Work out the finished part from the listing and answer in its coordinate system (mm). A direction names the side the tool comes from. Give positions to 0.01 mm unless a question says otherwise; leave off trailing zeros. Write each loop counter-clockwise with the first axis right and the second up, starting at its lowest first coordinate (ties: lowest second). Pieces come first, ordered by that corner, then holes. Notation, with made-up numbers: (-40, -35.5) -> (-7, -35.5) arc R15 ccw to (-7, -14.5) -> close; hole circle Ø3 at (-22.75, 25). An arc over 180 degrees is marked (long way). Write item = value, one per line. Start each with the question number.
from build123d import *

# Parameters (mm, degrees)
SKETCH1_W                      = 128
SKETCH1_H                      = 69
BOSS_EXTRUDE1_DEPTH            = 3
SKETCH5_R                      = 1.55
CUT_EXTRUDE5_DEPTH             = 10
SKETCH7_W                      = 28
SKETCH7_H                      = 8
BOSS_EXTRUDE2_DEPTH            = 5
SKETCH2_R                      = 2.05
CUT_EXTRUDE6_DEPTH             = 73.878323252
CUT_EXTRUDE6_DIRECTION_2_REACH = 74.878
CUT_EXTRUDE7_DEPTH             = 3
SKETCH8_W                      = 18
SKETCH8_H                      = 2
BOSS_EXTRUDE3_DEPTH            = 8
FILLET1_R                      = 3
FILLET2_R                      = 1


with BuildPart() as part:
    # Sketch1 → Boss-Extrude1 (new body)
    with BuildSketch(Plane(origin=(0, 0, 0), x_dir=(1, 0, 0), z_dir=(0, 1, 0))):
        Rectangle(SKETCH1_W, SKETCH1_H)
    extrude(amount=BOSS_EXTRUDE1_DEPTH)

    # Sketch5 → Cut-Extrude5 (cut)
    with BuildSketch(Plane(origin=(0, 3, 0), x_dir=(1, 0, 0), z_dir=(0, 1, 0))):
        with Locations(Location((0, -20.25, 0), (0, 0, 270))):
            Circle(SKETCH5_R)
        with Locations(Location((0, 20.25, 0), (0, 0, 270))):
            Circle(SKETCH5_R)
    extrude(amount=-CUT_EXTRUDE5_DEPTH, mode=Mode.SUBTRACT)

    # Sketch7 → Boss-Extrude2 (add)
    with BuildSketch(Plane(origin=(0, 3, 0), x_dir=(1, 0, 0), z_dir=(0, 1, 0))):
        with Locations((-50, 30.5)):
            Rectangle(SKETCH7_W, SKETCH7_H)
        with Locations((50, 30.5)):
            Rectangle(SKETCH7_W, SKETCH7_H)
        with Locations((50, -30.5)):
            Rectangle(SKETCH7_W, SKETCH7_H)
        with Locations((-50, -30.5)):
            Rectangle(SKETCH7_W, SKETCH7_H)
    extrude(amount=BOSS_EXTRUDE2_DEPTH)

    # Sketch2 → Cut-Extrude6 (cut)
    with BuildSketch(Plane(origin=(0, 3, 0), x_dir=(1, 0, 0), z_dir=(0, 1, 0))):
        with Locations(Location((-45, 30.5, 0), (0, 0, 270))):
            Circle(SKETCH2_R)
        with Locations(Location((45, 30.5, 0), (0, 0, 270))):
            Circle(SKETCH2_R)
        with Locations(Location((45, -30.5, 0), (0, 0, 270))):
            Circle(SKETCH2_R)
        with Locations(Location((-45, -30.5, 0), (0, 0, 270))):
            Circle(SKETCH2_R)
    extrude(amount=-CUT_EXTRUDE6_DEPTH, mode=Mode.SUBTRACT)

    # Sketch2 → Cut-Extrude6 direction 2 (cut, up to next)
    with BuildSketch(Plane(origin=(0, 3, 0), x_dir=(1, 0, 0), z_dir=(0, 1, 0)), mode=Mode.PRIVATE) as cut_extrude6_direction_2_sk1:
        with Locations(Location((-45, 30.5, 0), (0, 0, 270))):
            Circle(SKETCH2_R)
    cut_extrude6_direction_2_tool1 = extrude(cut_extrude6_direction_2_sk1.sketch, amount=CUT_EXTRUDE6_DIRECTION_2_REACH, mode=Mode.PRIVATE) & part.part
    # Sketch2 → Cut-Extrude6 direction 2 (cut, up to next)
    with BuildSketch(Plane(origin=(0, 3, 0), x_dir=(1, 0, 0), z_dir=(0, 1, 0)), mode=Mode.PRIVATE) as cut_extrude6_direction_2_sk2:
        with Locations(Location((45, 30.5, 0), (0, 0, 270))):
            Circle(SKETCH2_R)
    cut_extrude6_direction_2_tool2 = extrude(cut_extrude6_direction_2_sk2.sketch, amount=CUT_EXTRUDE6_DIRECTION_2_REACH, mode=Mode.PRIVATE) & part.part
    # Sketch2 → Cut-Extrude6 direction 2 (cut, up to next)
    with BuildSketch(Plane(origin=(0, 3, 0), x_dir=(1, 0, 0), z_dir=(0, 1, 0)), mode=Mode.PRIVATE) as cut_extrude6_direction_2_sk3:
        with Locations(Location((45, -30.5, 0), (0, 0, 270))):
            Circle(SKETCH2_R)
    cut_extrude6_direction_2_tool3 = extrude(cut_extrude6_direction_2_sk3.sketch, amount=CUT_EXTRUDE6_DIRECTION_2_REACH, mode=Mode.PRIVATE) & part.part
    # Sketch2 → Cut-Extrude6 direction 2 (cut, up to next)
    with BuildSketch(Plane(origin=(0, 3, 0), x_dir=(1, 0, 0), z_dir=(0, 1, 0)), mode=Mode.PRIVATE) as cut_extrude6_direction_2_sk4:
        with Locations(Location((-45, -30.5, 0), (0, 0, 270))):
            Circle(SKETCH2_R)
    cut_extrude6_direction_2_tool4 = extrude(cut_extrude6_direction_2_sk4.sketch, amount=CUT_EXTRUDE6_DIRECTION_2_REACH, mode=Mode.PRIVATE) & part.part
    add(cut_extrude6_direction_2_tool1.solids().sort_by_distance((-45, 3, -30.5))[0], mode=Mode.SUBTRACT)
    add(cut_extrude6_direction_2_tool2.solids().sort_by_distance((45, 3, -30.5))[0], mode=Mode.SUBTRACT)
    add(cut_extrude6_direction_2_tool3.solids().sort_by_distance((45, 3, 30.5))[0], mode=Mode.SUBTRACT)
    add(cut_extrude6_direction_2_tool4.solids().sort_by_distance((-45, 3, 30.5))[0], mode=Mode.SUBTRACT)

    # Sketch6 → Cut-Extrude7 (cut)
    with BuildSketch(Plane(origin=(0, 3, 0), x_dir=(1, 0, 0), z_dir=(0, 1, 0))):
        with BuildLine():
            Line((-45, 24.5), (-45, -24.5))
            add(Edge.make_bspline(
                [(-45, -24.5), (0.589986909, -9.997447075), (46.241142194, -24.5)],
                knots=[0, 0, 0, 1, 1, 1], degree=2))
            Line((46.241142194, -24.5), (46.241142194, 24.5))
            add(Edge.make_bspline(
                [(-45, 24.5), (0.589986909, 9.997447075), (46.241142194, 24.5)],
                knots=[0, 0, 0, 1, 1, 1], degree=2))
        make_face()
    extrude(amount=-CUT_EXTRUDE7_DEPTH, mode=Mode.SUBTRACT)

    # Sketch8 → Boss-Extrude3 (add)
    with BuildSketch(Plane(origin=(0, 3, 0), x_dir=(1, 0, 0), z_dir=(0, 1, 0))):
        with Locations((-45, 25.5)):
            Rectangle(SKETCH8_W, SKETCH8_H)
        with Locations((-45, -25.5)):
            Rectangle(SKETCH8_W, SKETCH8_H)
        with Locations((45, -25.5)):
            Rectangle(SKETCH8_W, SKETCH8_H)
        with Locations((45, 25.5)):
            Rectangle(SKETCH8_W, SKETCH8_H)
    extrude(amount=BOSS_EXTRUDE3_DEPTH)

    # Fillet1
    fillet1_edges = [part.edges().sort_by_distance(p)[0] for p in [
        (64, 4, 34.5),
        (-64, 4, 34.5),
        (-64, 4, -34.5),
        (64, 4, -34.5),
    ]]
    fillet(fillet1_edges, radius=FILLET1_R)

    # Fillet2
    fillet2_edges = [part.edges().sort_by_distance(p)[0] for p in [
        (64, 8, -29),
        (63.121320344, 8, -33.621320344),
        (48.5, 8, -34.5),
        (36, 5.5, -34.5),
        (45, 11, -24.5),
        (45, 11, -26.5),
        (45, 11, 26.5),
        (45, 11, 24.5),
        (-45, 11, 26.5),
        (-45, 11, 24.5),
        (-45, 11, -24.5),
        (-45, 11, -26.5),
        (-64, 8, -29),
        (-63.121320344, 8, -33.621320344),
        (-64, 8, 29),
        (-63.121320344, 8, 33.621320344),
        (48.5, 8, 34.5),
        (63.121320344, 8, 33.621320344),
        (-48.5, 8, -34.5),
        (-48.5, 8, 34.5),
        (-36, 9.5, 26.5),
        (54, 9.5, 26.5),
        (64, 8, 29),
    ]]
    fillet(fillet2_edges, radius=FILLET2_R - 0.0001)  # a hair under: the kernel refuses the full size


solid = part.part
(1) A cutting plane is placed at B-B, the plane z = 7.5. Write down the section's boundary in (x, y), then the cut area to 3 significant figures.
(2) Each of these flat-tipped pins is pushed along its axis until it touches: pin 1 (14 mm diameter, centred on x = 54, z = -10, fed in from +Y); pin 2 (0.6 mm diameter, centred on x = -46, y = 9, fed in from -Z); pin 3 (5.5 mm diameter, centred on x = -53.5, z = -30, fed in from +Y); pin 4 (5 mm diameter, centred on x = 25, z = 15, fed in from -Y). Where does it stop, or does it pass through?
(3) Find the intervals of material crossed by line 1 along X through (y, z) = (6.25, 30.5); line 2 along X through (y, z) = (1.5, 30.5); line 3 along Z through (x, y) = (-45, 6), in increasing order.
(4) For faces 4 (the flat face through (-59, 5, 26.5)), 5 (the flat face through (-36, 6, 30)), 6 (the flat face through (59, 5, -26.5)), 7 (the flat face through (46.241, 2, 0)), 8 (the flat face through (45, 6, -24.5)), determine the directions among +Z, -Z, +X, -X, +Y, -Y from which every point of the face is accessible in a straight line to the end or side of a thin tool.
(5) A cutting plane is placed at A-A, the plane y = 5.25. State how many separate pieces and enclosed holes the cut face has, then the cut area to 3 significant figures.
(6) Determine the mould class of faces 1 (the flat face through (49, 8, -30)), 2 (the cylindrical face through (63.14, 3.55, 33.6)), 3 (the cylindrical face through (-42.967, 4.056, 30.233)) for opening direction X: pulls with the +X half, pulls with the -X half, needs draft (parallel to the pull), parting line crosses it, or undercut.
Results list:
q1.outline = (-64, 0) -> (-45, 0) -> (-45, 3) -> (-64, 3) -> close; (46.24, 0) -> (64, 0) -> (64, 3) -> (46.24, 3) -> close
q1.area = 110 mm²
q2.pin_1 = 3
q2.pin_2 = -26.5
q2.pin_3 = 8
q2.pin_4 = through
q3.line_1 = -64 to -47.05, -42.95 to -36, 36 to 42.95, 47.05 to 64
q3.line_2 = -64 to -47.05, -42.95 to 42.95, 47.05 to 64
q3.line_3 = -34.5 to -32.55, -28.45 to -24.5, 24.5 to 28.45, 32.55 to 34.5
q4.face_4 = -X, +Y
q4.face_5 = +Z, -Z, +Y
q4.face_6 = +X, +Y
q4.face_7 = +Y, -Y
q4.face_8 = +X, -X, +Y
q5.separate_pieces = 4
q5.enclosed_holes = 4
q5.area = 979 mm²
q6.face_1 = needs draft
q6.face_2 = pulls with the +X half
q6.face_3 = undercut
